```python
from build123d import *

# Parameters (mm, degrees)
F2_R     = 15.24
F3_DEPTH = 30.48


with BuildPart() as f1:
    # F0 (on Front) → F1 (revolve)
    with BuildSketch(Plane.XZ):
        Polygon((0, 30.48), (0, 0), (30.48, 0), align=None)
    revolve(axis=Axis((0, 0, 15.24), (0, 0, 1)))


with BuildPart() as f3:
    # F2 (on Top) → F3 (new body)
    with BuildSketch(Plane.XY):
        with Locations((-47.422264, -15.657526)):
            Circle(F2_R)
    extrude(amount=F3_DEPTH)


solid = f1.part
```
For this review, take the finished solid that the model builds, in its own axes (mm). Coordinates: 2 decimals unless noted, no trailing zeros. Order: outer loops, then holes, each group sorted by start corner. A loop starts at its lowest first (then second) coordinate and runs counter-clockwise, first axis right, second up. Notation, with made-up numbers: (50.25, 62) - (73.25, 62) arc R23 ccw to (73.25, 78) - close; hole circle Ø8 at (40.25, 72.5). An arc over 180 degrees is marked (long way). Answer as a JSON object with one key per item and string values. Group by question number.
1. For probe 1 along Y at (x, z) = (2.5, 15.5); probe 2 along Z at (x, y) = (26.5, 11); probe 3 along Y at (x, z) = (19, 2), list the stretches that pass through material, from the lowest coordinate up.
2. We need section B-B on z = 9. State the section outline as (x, y) points, then the cut area to 3 significant figures.
3. We need section A-A on z = 14. State the section outline as (x, y) points, then the cut area to 3 significant figures.
4. Clearance check with flat-ended pins moving along their axes: P1, Ø4, axis at x = 9.5, y = 14, coming from the -Z side; P2, Ø12, axis at x = 8, z = 15.5, coming from the -Y side; P3, Ø6, axis at x = -2.5, y = 7.5, coming from the +Z side; P4, Ø1, axis at y = -9, z = 23.5, coming from the -X side. State where each tip first meets the part, or that it passes through.
Final values:
{
 "1": {"probe 1": "-14.77 to 14.77", "probe 2": "0 to 1.79", "probe 3": "-21.22 to 21.22"},
 "2": {"outline": "circle Ø42.96 at (0, 0)", "area": "1,450 mm²"},
 "3": {"outline": "circle Ø32.96 at (0, 0)", "area": "853 mm²"},
 "4": {"P1": "z = 0", "P2": "y = -19.75", "P3": "z = 25.57", "P4": "through"}
}
